```python
from build123d import *

# Parameters (mm, degrees)
SKETCH1_R                      = 69.85
BOSS_EXTRUDE1_DEPTH            = 3.81
SKETCH4_R                      = 25.4
BOSS_EXTRUDE5_DEPTH            = 7.99999997
SKETCH25_R                     = 11.43
CUT_EXTRUDE4_DEPTH             = 3.99999997
SKETCH5_R                      = 6
BOSS_EXTRUDE6_DEPTH            = 0.508
SKETCH26_R                     = 3.95
BOSS_EXTRUDE7_DEPTH            = 5
CUT_EXTRUDE1_DEPTH             = 100.486285986
CUT_EXTRUDE1_DEPTH_BACK        = 100.486285986
SKETCH6_R                      = 2.5
TAP_DRILL_FOR_M1_2X0_25_TAP1_D = 28.3


with BuildPart() as part:
    # Sketch1 → Boss-Extrude1 (new body)
    with BuildSketch(Plane(origin=(0, 0, 0), x_dir=(1, 0, 0), z_dir=(0, 1, 0))):
        with Locations(Location((0, 0, 0), (0, 0, 90))):
            Circle(SKETCH1_R)
    extrude(amount=BOSS_EXTRUDE1_DEPTH)

    # Sketch4 → Boss-Extrude5 (add)
    with BuildSketch(Plane(origin=(0, 3.81, 0), x_dir=(1, 0, 0), z_dir=(0, 1, 0))):
        with Locations(Location((0, 0, 0), (0, 0, 270))):
            Circle(SKETCH4_R)
    extrude(amount=BOSS_EXTRUDE5_DEPTH)

    # Sketch25 → Cut-Extrude4 (cut)
    with BuildSketch(Plane.XZ):
        with Locations(Location((0, 0, 0), (0, 0, 270))):
            Circle(SKETCH25_R)
    extrude(amount=-CUT_EXTRUDE4_DEPTH, mode=Mode.SUBTRACT)

    # Sketch5 → Boss-Extrude6 (add)
    with BuildSketch(Plane(origin=(0, 3.99999997, 0), x_dir=(1, 0, 0), z_dir=(0, 1, 0))):
        with Locations(Location((0, 0, 0), (0, 0, 270))):
            Circle(SKETCH5_R)
    extrude(amount=-BOSS_EXTRUDE6_DEPTH)

    # Sketch26 → Boss-Extrude7 (add)
    with BuildSketch(Plane.XZ.offset(-3.49199997)):
        with Locations(Location((0, 0, 0), (0, 0, 270))):
            Circle(SKETCH26_R)
    extrude(amount=BOSS_EXTRUDE7_DEPTH)

    # Sketch6 → Cut-Extrude1 (cut, two sides: drawn at the far end of the back side and taken through both)
    with BuildSketch(Plane.XZ.offset(-CUT_EXTRUDE1_DEPTH_BACK)):
        with Locations(Location((0, 0, 0), (0, 0, 270))):
            Circle(SKETCH6_R)
    extrude(amount=CUT_EXTRUDE1_DEPTH + CUT_EXTRUDE1_DEPTH_BACK, mode=Mode.SUBTRACT)

    # Tap Drill for M1.2x0.25 Tap1 (through all)
    with Locations(Plane(origin=(0, 3.81, 0), x_dir=(1, 0, 0), z_dir=(0, 1, 0))):
        with Locations((-50.8, 0), (-41.098063314, 29.859490816), (-15.698063314, 48.313671028), (15.698063314, 48.313671028), (41.098063314, 29.859490816), (50.8, 0), (41.098063314, -29.859490816), (15.698063314, -48.313671028), (-15.698063314, -48.313671028), (-41.098063314, -29.859490816)):
            Hole(TAP_DRILL_FOR_M1_2X0_25_TAP1_D / 2)


solid = part.part
```
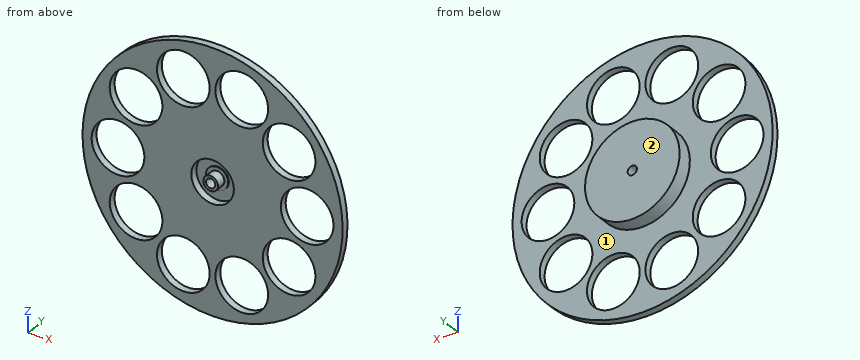
The listing builds one solid part. Answer for the finished solid, in the listing's coordinates (mm). Face numbers are marked on the shaded views. A direction names the side the tool comes from. Give positions to 0.01 mm unless a question says otherwise; leave off trailing zeros. Order: outer loops, then holes, each group sorted by start corner. A loop starts at its lowest first (then second) coordinate and runs counter-clockwise, first axis right, second up. Notation, with made-up numbers: (5, 70) -> (9, 70) arc R6 ccw to (9, 80) -> close; hole circle Ø5 at (-2, 26.5). An arc over 180 degrees is marked (long way). Answer as CSV lines item,"result". Start each with the question number.
Q1. A cutting plane is placed at B-B (x = -15.5). Determine the outline of the cut face in (y, z), then the cut area to 3 significant figures.
Q2. Given pin 1 (1 mm diameter, centred on y = 4, z = -18.5, fed in from -X); pin 2 (5 mm diameter, centred on x = 11.5, z = -32.5, fed in from -Y); pin 3 (3 mm diameter, centred on x = 0, z = 0, fed in from +Y); pin 4 (6 mm diameter, centred on x = 39, y = 3, fed in from -Z), each flat-ended and moving along its own axis, determine where each tip first touches the part or whether it passes through.
Q3. A cutting plane is placed at D-D (x = 60). Determine the outline of the cut face in (y, z).
Q4. Find the intervals of material crossed by L1, parallel to X at y = 2.25, z = -17; L2, parallel to X at y = 2.25, z = -6; L3, parallel to X at y = 5.5, z = 0, in increasing order.
Q5. A cutting plane is placed at A-A (z = 0). Count the separate pieces of the cut face and the enclosed holes in it, then the cut area to 3 significant figures.
Q6. Which of the six approach directions +Z, -Z, +X, -X, +Y, -Y give full straight-line access (tool end or side, diameter ignored) to the marked faces 1 and 2?
Q7. A cutting plane is placed at C-C (y = 9.25). Determine the outline of the cut face in (x, z).
Results found:
1,outline,"(0, -68.11) -> (3.81, -68.11) -> (3.81, -62.46) -> (0, -62.46) -> close; (0, -34.17) -> (3.81, -34.17) -> (3.81, -20.12) -> (11.81, -20.12) -> (11.81, 20.12) -> (3.81, 20.12) -> (3.81, 34.17) -> (0, 34.17) -> close; (0, 62.46) -> (3.81, 62.46) -> (3.81, 68.11) -> (0, 68.11) -> close"
1,area,"625 mm2"
2,pin 1,"x = -67.48"
2,pin 2,"y = 0"
2,pin 3,"through"
2,pin 4,"z = -59.86"
3,outline,"(0, -35.76) -> (3.81, -35.76) -> (3.81, -10.75) -> (0, -10.75) -> close; (0, 10.75) -> (3.81, 10.75) -> (3.81, 35.76) -> (0, 35.76) -> close"
4,L1,"-67.75 to -47, -35.19 to 35.19, 47 to 67.75"
4,L2,"-69.59 to -63.61, -37.99 to -9.73, 9.73 to 37.99, 63.61 to 69.59"
4,L3,"-25.4 to -2.5, 2.5 to 25.4"
5,separate pieces,"4"
5,enclosed holes,"0"
5,area,"611 mm2"
6,face 1,"+Y"
6,face 2,"+Z, -Z, +X, -X, +Y"
7,outline,"circle Ø50.8 at (0, 0); hole circle Ø5 at (0, 0)"
